```python
from build123d import *

# Parameters (mm, degrees)
EXTRUDE_1_DEPTH       = 30
HOLE_WIZARD_M35_D     = 3.15
HOLE_WIZARD_M35_DEPTH = 8
HOLE_WIZARD_M35_TIP   = 0.946355475
HOLE_WIZARD_M36_D     = 3.15
HOLE_WIZARD_M36_DEPTH = 8
HOLE_WIZARD_M36_TIP   = 0.946355475


with BuildPart() as part:
    # Эскиз1 → Бобышка-Вытянуть1 (new body)
    with BuildSketch(Plane(origin=(0, 0, 0), x_dir=(1, 0, 0), z_dir=(0, 1, 0))):
        Polygon((2.886751346, 0), (1.443375673, 2.5), (-1.443375673, 2.5), (-2.886751346, 0), (-1.443375673, -2.5), (1.443375673, -2.5), align=None)
    extrude(amount=EXTRUDE_1_DEPTH)

    # Сверло под метчик  спиральное M35
    with Locations(Plane(origin=(0, 30, 0), x_dir=(1, 0, 0), z_dir=(0, 1, 0))):
        with Locations((0, 0)):
            Hole(HOLE_WIZARD_M35_D / 2, depth=HOLE_WIZARD_M35_DEPTH)
            with Locations((0, 0, -(HOLE_WIZARD_M35_DEPTH + HOLE_WIZARD_M35_TIP / 2))):  # 118° drill point
                Cone(0, HOLE_WIZARD_M35_D / 2, HOLE_WIZARD_M35_TIP, mode=Mode.SUBTRACT)

    # Сверло под метчик  спиральное M36
    with Locations(Plane(origin=(0, 0, 0), x_dir=(-1, 0, 0), z_dir=(0, -1, 0))):
        with Locations((0, 0)):
            Hole(HOLE_WIZARD_M36_D / 2, depth=HOLE_WIZARD_M36_DEPTH)
            with Locations((0, 0, -(HOLE_WIZARD_M36_DEPTH + HOLE_WIZARD_M36_TIP / 2))):  # 118° drill point
                Cone(0, HOLE_WIZARD_M36_D / 2, HOLE_WIZARD_M36_TIP, mode=Mode.SUBTRACT)


solid = part.part
```
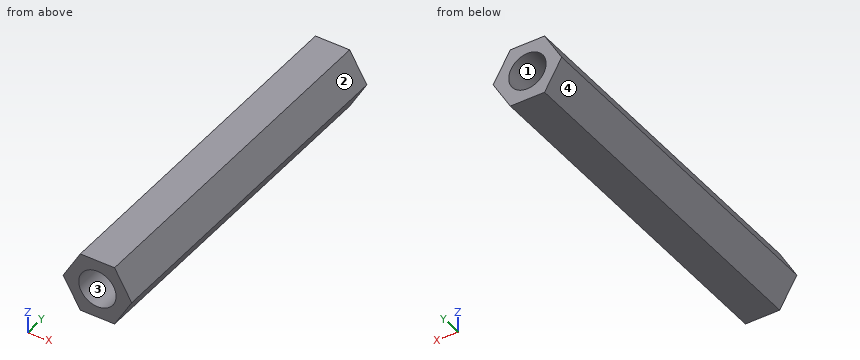
Part model, mm, in its own coordinate system. Face numbers are marked on the shaded views. Round coordinates to 2 decimals unless told otherwise and drop trailing zeros. Loops run counter-clockwise (first coordinate to the right, second up) from the corner with the lowest first, then second, coordinate; pieces in that order, holes last.
Item 1: Mould opens along X. For the marked faces 1, 2, 3 and 4 say: +X half, -X half, draft (parallel to the pull), parting line (faces both ways), or undercut.
Item 2: Cut at D-D, the plane z = 2.1. Give the cut face in (x, y), then the cut area to 3 significant figures.
Item 3: Cut at B-B, the plane y = 12. Give the cut face in (x, z).
Item 4: Drop a flat-ended pin along its axis: P1, Ø2.5, axis at x = 0, z = 0, coming from the +Y side. Give the stop position or say it passes through.
Item 5: Cut at C-C, the plane x = -2.3. Give the cut face in (y, z), then the cut area to 3 significant figures.
Item 6: Drill centre lines: line 1 (Z direction, x = 0, y = 25.25) (3 decimals); line 2 (Z direction, x = -2.05, y = 12.5); line 3 (X direction, y = 23.25, z = -0.15). Where is each one in solid material? Low to high.
Item 7: Cut at A-A, the plane y = 2.5. Give the cut face in (x, z) (3 decimals).
A:
1. face 1: undercut
1. face 2: +X half
1. face 3: undercut
1. face 4: -X half
2. outline: (-1.67, 0) - (1.67, 0) - (1.67, 30) - (-1.67, 30) - close
2. area: 100 mm2
3. outline: (-2.89, 0) - (-1.44, -2.5) - (1.44, -2.5) - (2.89, 0) - (1.44, 2.5) - (-1.44, 2.5) - close
4. P1: stops at y = 21.8
5. outline: (0, -1.02) - (30, -1.02) - (30, 1.02) - (0, 1.02) - close
5. area: 61.0 mm2
6. line 1: z = -2.5 to -1.575, 1.575 to 2.5
6. line 2: z = -1.45 to 1.45
6. line 3: x = -2.8 to -1.57, 1.57 to 2.8
7. outline: (-2.887, 0) - (-1.443, -2.5) - (1.443, -2.5) - (2.887, 0) - (1.443, 2.5) - (-1.443, 2.5) - close; hole circle Ø3.15 at (0, 0)
